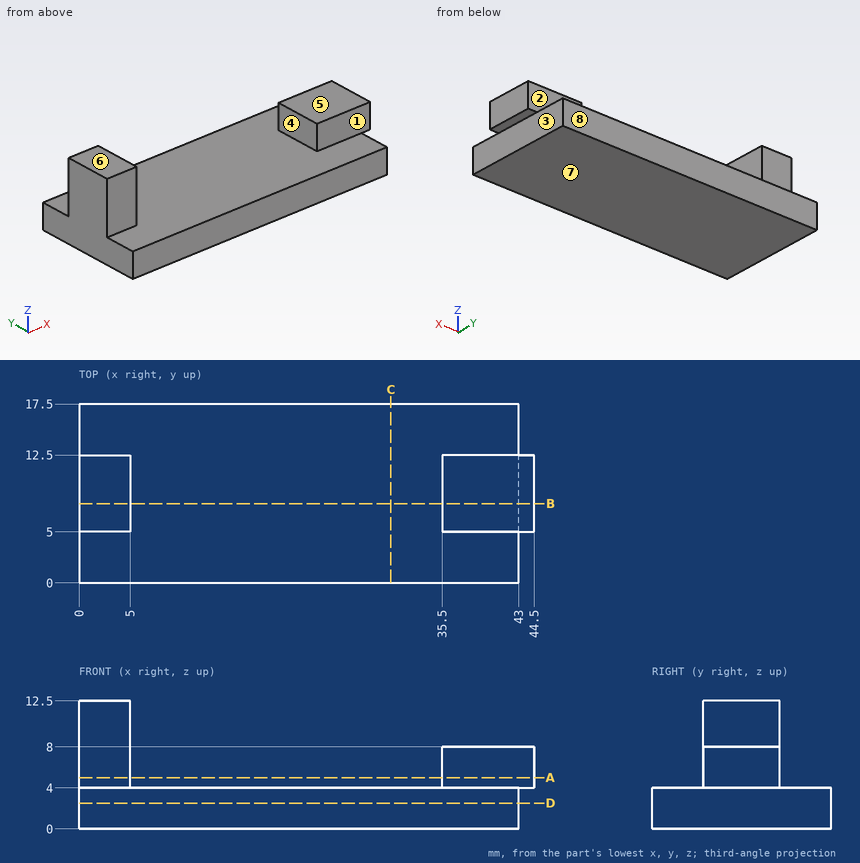
Here's the drawing with two shaded views (mm, measured from the low corner). I have some questions. A direction names the side the tool comes from. Give positions to 0.01 mm unless a question says otherwise; leave off trailing zeros. Order: outer loops, then holes, each group sorted by start corner. A loop starts at its lowest first (then second) coordinate and runs counter-clockwise, first axis right, second up. Notation, with made-up numbers: (18.5, 84) - (58.5, 84) arc R15 ccw to (58.5, 106) - close; hole circle Ø7 at (47.25, 14). An arc over 180 degrees is marked (long way). Use a Markdown table: item, result. Add a question column.
Q1. If we section it at D-D on z = 2.5: Write out the boundary of the cut face in (x, y).
Q2. Please list where these lines run through material, in increasing order: line 1 along X through (y, z) = (11.5, 7); line 2 along Z through (x, y) = (29.5, 2.25); line 3 along Z through (x, y) = (38, 8.5).
Q3. On a 3-axis mill with a long thin cutter (end or side, diameter ignored), from which of +Z, -Z, +X, -X, +Y, -Y can I reach the whole of each face in a straight line? I mean the marked faces 1, 2, 3, 4 and 5. Say none if no direction works.
Q4. I'm going to push flat-ended pins straight in: pin 1 (5 mm diameter, centred on x = 18, y = 10.5, fed in from +Z); pin 2 (8 mm diameter, centred on x = 41, y = 10.5, fed in from +Z); pin 3 (4 mm diameter, centred on x = 3.5, z = 6.5, fed in from -Y). Where does each tip first touch, or does it pass through?
Q5. If we section it at B-B on y = 7.75: Write out the boundary of the cut face in (x, z).
Q6. If we section it at A-A on z = 5: Write out the boundary of the cut face in (x, y).
Q7. If we section it at C-C on x = 30.5: Write out the boundary of the cut face in (y, z), plus the area to 3 significant figures.
Q8. If we mould it in two halves opening along Z, with no side actions, what happens to the marked faces 6, 7 and 8? For each: released by +Z, released by -Z, zero draft, split by the parting line, or undercut.
Answers follow:
| question | item | result |
|---|---|---|
| 1 | outline | (0, 0) - (43, 0) - (43, 17.5) - (0, 17.5) - close |
| 2 | line 1 | x = 0 to 5, 35.5 to 44.5 |
| 2 | line 2 | z = 0 to 4 |
| 2 | line 3 | z = 0 to 8 |
| 3 | face 1 | +Z, +X, -X, -Y |
| 3 | face 2 | +Z, +X, -X, +Y |
| 3 | face 3 | -Z, +X, +Y, -Y |
| 3 | face 4 | +Z, +Y, -Y |
| 3 | face 5 | +Z, +X, +Y, -Y |
| 4 | pin 1 | stops at z = 4 |
| 4 | pin 2 | stops at z = 8 |
| 4 | pin 3 | stops at y = 5 |
| 5 | outline | (0, 0) - (43, 0) - (43, 4) - (44.5, 4) - (44.5, 8) - (35.5, 8) - (35.5, 4) - (5, 4) - (5, 12.5) - (0, 12.5) - close |
| 6 | outline | (0, 5) - (5, 5) - (5, 12.5) - (0, 12.5) - close; (35.5, 5) - (44.5, 5) - (44.5, 12.5) - (35.5, 12.5) - close |
| 7 | outline | (0, 0) - (17.5, 0) - (17.5, 4) - (0, 4) - close |
| 7 | area | 70.0 mm^2 |
| 8 | face 6 | released by +Z |
| 8 | face 7 | released by -Z |
| 8 | face 8 | zero draft |
